Check sheet for the modelled part. Datum: model origin and axes. Units: mm. Give positions to 0.01 mm unless a question says otherwise; leave off trailing zeros. Loops run counter-clockwise (first coordinate to the right, second up) from the corner with the lowest first, then second, coordinate; pieces in that order, holes last. Notation, with made-up numbers: (53, 84) - (61, 84) arc R23 ccw to (61, 109) - close; hole circle Ø2 at (11.25, -5). An arc over 180 degrees is marked (long way). Answer in a Markdown table with one row per item. Add a question column.
(1) Sectioned sample at A-A on x = 0. Enter the section's corners in (y, z).
(2) Go/stop test with flat-tipped pins: P1, Ø1, axis at x = 3.5, z = -0.5, coming from the +Y side; P2, Ø1, axis at y = -2, z = 0.5, coming from the +X side. Record where each tip stops, or that it passes through.
(3) Draft check along X on faces 1 (the face through (4.88, -1.08, 0.01)), 2 (the face through (5.5, 0, -1)), 3 (the face through (2.681, 6.466, 0.01)). Enter one of: released by +X, released by -X, zero draft, split by the parting line, or undercut.
(4) Thickness scan on L1, parallel to X at y = 0, z = 0.4; L2, parallel to Y at x = -4.5, z = -0.5. Record the ranges inside material, lowest first.
(5) Sectioned sample at C-C on z = -0.45. Enter the section's corners in (x, y), then the cut area to 3 significant figures.
from build123d import *

# Parameters (mm, degrees)
F1_W = 2
F1_H = 2
F3_R = 0.25


with BuildPart() as f2:
    # F1 (on Right) → F2 (revolve)
    with BuildSketch(Plane.YZ):
        with Locations((6, 0)):
            Rectangle(F1_W, F1_H)
    revolve(axis=Axis((0, 0, 8.067548), (0, 0, 1)))

    # F3
    f3_edges = [f2.edges().sort_by_distance(p)[0] for p in [
        (0, -7, 1),
        (0, -5, 1),
        (0, -7, -1),
        (0, -5, -1),
    ]]
    fillet(f3_edges, radius=F3_R)


solid = f2.part
Reply:
| question | item | result |
|---|---|---|
| 1 | outline | (-7, -0.75) arc R0.25 ccw to (-6.75, -1) - (-5.25, -1) arc R0.25 ccw to (-5, -0.75) - (-5, 0.75) arc R0.25 ccw to (-5.25, 1) - (-6.75, 1) arc R0.25 ccw to (-7, 0.75) - close; (5, -0.75) arc R0.25 ccw to (5.25, -1) - (6.75, -1) arc R0.25 ccw to (7, -0.75) - (7, 0.75) arc R0.25 ccw to (6.75, 1) - (5.25, 1) arc R0.25 ccw to (5, 0.75) - close |
| 2 | P1 | y = 6.32 |
| 2 | P2 | x = 6.84 |
| 3 | face 1 | undercut |
| 3 | face 2 | zero draft |
| 3 | face 3 | split by the parting line |
| 4 | L1 | -7 to -5, 5 to 7 |
| 4 | L2 | -5.36 to -2.18, 2.18 to 5.36 |
| 5 | outline | circle Ø14 at (0, 0); hole circle Ø10 at (0, 0) |
| 5 | area | 75.4 mm^2 |
